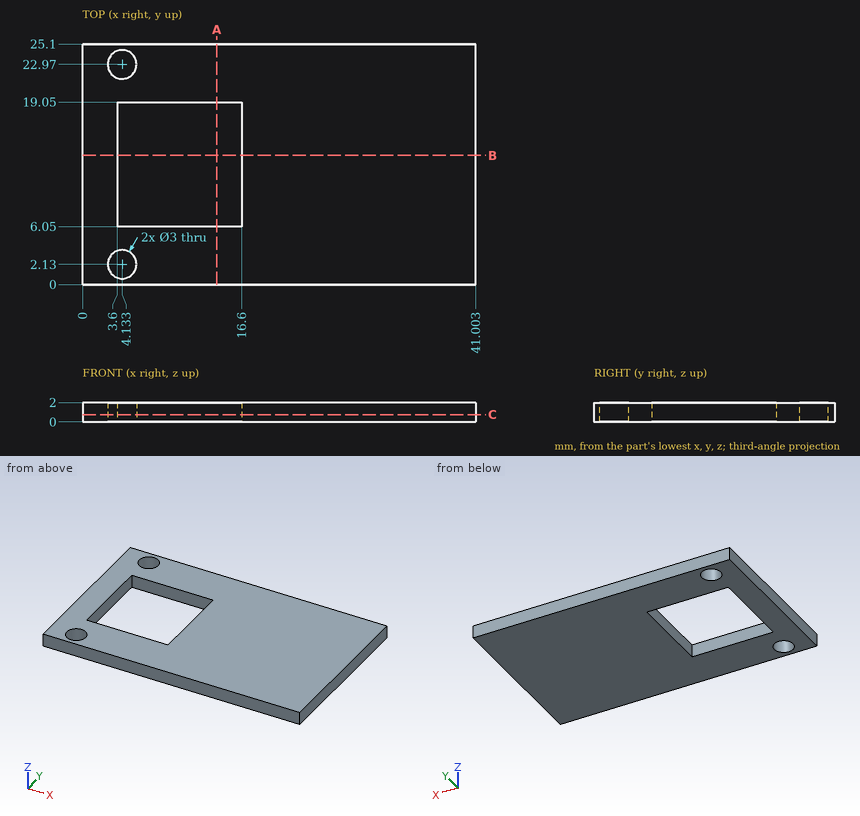
Answer from the drawing. Dimensions are ordinates in mm from the lowest x, y and z of the part. Coordinates: 2 decimals unless noted, no trailing zeros. Loops run counter-clockwise (first coordinate to the right, second up) from the corner with the lowest first, then second, coordinate; pieces in that order, holes last. Notation, with made-up numbers: (27.5, -3.75) -> (57.5, -3.75) arc R9 ccw to (57.5, 6.25) -> close; hole circle Ø8 at (-20, 15.5). An arc over 180 degrees is marked (long way). Return JSON: item names as keys, results as strings.
Item 1: Find section A-A (x = 14). Determine the outline of the cut face in (y, z).
Answers:
{"outline": "(0, 0) -> (6.05, 0) -> (6.05, 2) -> (0, 2) -> close; (19.05, 0) -> (25.1, 0) -> (25.1, 2) -> (19.05, 2) -> close"}
Item 2: Find section B-B (y = 13.5). Determine the outline of the cut face in (x, z).
Answers:
{"outline": "(0, 0) -> (3.6, 0) -> (3.6, 2) -> (0, 2) -> close; (16.6, 0) -> (41, 0) -> (41, 2) -> (16.6, 2) -> close"}
Item 3: Find section C-C (z = 0.75). Determine the outline of the cut face in (x, y), plus the area to 3 significant figures.
Answers:
{"outline": "(0, 0) -> (41, 0) -> (41, 25.1) -> (0, 25.1) -> close; hole circle Ø3 at (4.13, 2.13); hole circle Ø3 at (4.13, 22.97); hole (3.6, 6.05) -> (16.6, 6.05) -> (16.6, 19.05) -> (3.6, 19.05) -> close", "area": "846 mm2"}
Item 4: Find the intervals of material crossed by probe 1 along X at (y, z) = (2.13, 0.4); probe 2 along X at (y, z) = (11.5, 1.4); probe 3 along Y at (x, z) = (12, 0.85), in increasing order.
Answers:
{"probe 1": "x = 0 to 2.63, 5.63 to 41", "probe 2": "x = 0 to 3.6, 16.6 to 41", "probe 3": "y = 0 to 6.05, 19.05 to 25.1"}
Item 5: A flat-ended cylindrical pin translates along its axis: P1, Ø4, axis at x = 4.13, y = 2.13, coming from the +Z side. Find the tip coordinate at first contact, or state that the pin passes through.
Answers:
{"P1": "stops at z = 2"}
